```python
from build123d import *

# Parameters (mm, degrees)
SKETCH2_R           = 36.6
SKETCH2_R_2         = 29.45
BOSS_EXTRUDE1_DEPTH = 140
SKETCH3_R           = 36.6
BOSS_EXTRUDE2_DEPTH = 15
SKETCH5_R           = 3.175
CUT_EXTRUDE1_DEPTH  = 52
SKETCH6_R           = 4
SKETCH6_R_2         = 3.175
BOSS_EXTRUDE4_DEPTH = 52
SKETCH7_R           = 3.175
CUT_EXTRUDE2_DEPTH  = 52
SKETCH8_R           = 4
SKETCH8_R_2         = 3.175
BOSS_EXTRUDE5_DEPTH = 10
SKETCH4_R           = 36.6
BOSS_EXTRUDE3_DEPTH = 15


with BuildPart() as part:
    # Sketch2 → Boss-Extrude1 (new body, symmetric)
    with BuildSketch(Plane(origin=(0, 0, 0), x_dir=(1, 0, 0), z_dir=(0, 1, 0))):
        Circle(SKETCH2_R)
        Circle(SKETCH2_R_2, mode=Mode.SUBTRACT)
    extrude(amount=BOSS_EXTRUDE1_DEPTH, both=True)

    # Sketch3 → Boss-Extrude2 (add)
    with BuildSketch(Plane(origin=(0, 140, 0), x_dir=(1, 0, 0), z_dir=(0, 1, 0))):
        Circle(SKETCH3_R)
    extrude(amount=BOSS_EXTRUDE2_DEPTH)

    # Sketch5 → Cut-Extrude1 (cut)
    with BuildSketch(Plane.XY):
        with Locations((0, -117.704465643)):
            Circle(SKETCH5_R)
    extrude(amount=CUT_EXTRUDE1_DEPTH, mode=Mode.SUBTRACT)

    # Sketch6 → Boss-Extrude4 (add)
    with BuildSketch(Plane.XY):
        with Locations((0, -117.704465643)):
            Circle(SKETCH6_R)
        with Locations((0, -117.704465643)):
            Circle(SKETCH6_R_2, mode=Mode.SUBTRACT)
    extrude(amount=BOSS_EXTRUDE4_DEPTH)

    # Sketch7 → Cut-Extrude2 (cut)
    with BuildSketch(Plane(origin=(0, 155, 0), x_dir=(1, 0, 0), z_dir=(0, 1, 0))):
        with Locations((0, 20)):
            Circle(SKETCH7_R)
        Circle(SKETCH7_R)
        with Locations((-20, 0)):
            Circle(SKETCH7_R)
        with Locations((20, 0)):
            Circle(SKETCH7_R)
        with Locations((0, -20)):
            Circle(SKETCH7_R)
    extrude(amount=-CUT_EXTRUDE2_DEPTH, mode=Mode.SUBTRACT)

    # Sketch8 → Boss-Extrude5 (add)
    with BuildSketch(Plane(origin=(0, 155, 0), x_dir=(1, 0, 0), z_dir=(0, 1, 0))):
        Circle(SKETCH8_R)
        Circle(SKETCH8_R_2, mode=Mode.SUBTRACT)
        with Locations((0, 20)):
            Circle(SKETCH8_R)
        with Locations((0, 20)):
            Circle(SKETCH8_R_2, mode=Mode.SUBTRACT)
        with Locations((20, 0)):
            Circle(SKETCH8_R)
        with Locations((20, 0)):
            Circle(SKETCH8_R_2, mode=Mode.SUBTRACT)
        with Locations((-20, 0)):
            Circle(SKETCH8_R)
        with Locations((-20, 0)):
            Circle(SKETCH8_R_2, mode=Mode.SUBTRACT)
        with Locations((0, -20)):
            Circle(SKETCH8_R)
        with Locations((0, -20)):
            Circle(SKETCH8_R_2, mode=Mode.SUBTRACT)
    extrude(amount=BOSS_EXTRUDE5_DEPTH)

    # Sketch4 → Boss-Extrude3 (add)
    with BuildSketch(Plane.XZ.offset(140)):
        Circle(SKETCH4_R)
    extrude(amount=BOSS_EXTRUDE3_DEPTH)


solid = part.part
```
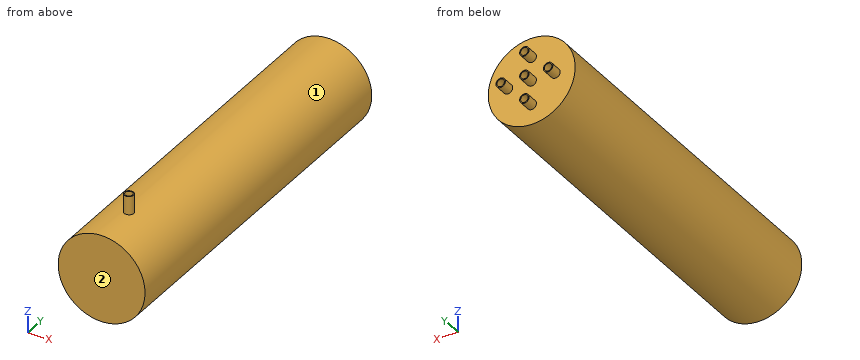
CAD build for the part. Positions are in the model's coordinates, mm. Face numbers are marked on the shaded views. Round coordinates to 2 decimals unless told otherwise and drop trailing zeros. Write each loop counter-clockwise with the first axis right and the second up, starting at its lowest first coordinate (ties: lowest second). Pieces come first, ordered by that corner, then holes. Notation, with made-up numbers: (10.5, -27.5) - (69.5, -27.5) arc R7 ccw to (69.5, -15.5) - close; hole circle Ø10 at (-39, -40). An arc over 180 degrees is marked (long way). Return JSON: item names as keys, results as strings. Group by question number.
Item 1: Probe probe 1 along Z at (x, y) = (0, 151) (3 decimals); probe 2 along Y at (x, z) = (17, 18); probe 3 along Z at (x, y) = (0, 159.5) (3 decimals). List the from-to ranges inside material, lowest first.
Item 2: Mould opens along X. For the marked faces 1 and 2 say: +X half, -X half, draft (parallel to the pull), parting line (faces both ways), or undercut.
Item 3: Band-saw the part on A-A on z = 10. List the corners of the cut face in (x, y) (3 decimals), plus the area to 3 significant figures.
Item 4: Flat gauge pins, fed straight in: pin 1 Ø1 at (x, y) = (17, 41) entering from -Z; pin 2 Ø9 at (x, y) = (-0.5, -118) entering from -Z; pin 3 Ø1 at (x, z) = (16.5, -16.5) entering from +Y. Where does each tip first touch, or does it go through?
Item 5: Band-saw the part on D-D on z = -20. List the corners of the cut face in (x, y) (3 decimals).
Item 6: Band-saw the part on C-C on y = -20.5. List the corners of the cut face in (x, z), plus the area to 3 significant figures.
Item 7: Band-saw the part on B-B on x = -20. List the corners of the cut face in (y, z) (3 decimals), plus the area to 3 significant figures.
Resolved:
{
 "1": {"probe 1": "z = -36.6 to -23.175, -16.825 to -3.175, 3.175 to 16.825, 23.175 to 36.6", "probe 2": "y = -155 to -140, 140 to 155", "probe 3": "z = -24 to -23.175, -16.825 to -16, -4 to -3.175, 3.175 to 4, 16 to 16.825, 23.175 to 24"},
 "2": {"face 1": "parting line", "face 2": "draft"},
 "3": {"outline": "(-35.207, -155) - (35.207, -155) - (35.207, 155) - (-35.207, 155) - close; circle Ø8 at (0, -117.704); hole (-27.7, -140) - (27.7, -140) - (27.7, 140) - (-27.7, 140) - close; hole circle Ø6.35 at (0, -117.704)", "area": "6,340 mm²"},
 "4": {"pin 1": "stops at z = -32.67", "pin 2": "stops at z = -36.6", "pin 3": "stops at y = 155"},
 "5": {"outline": "(-30.652, -155) - (30.652, -155) - (30.652, 155) - (4, 155) - (4, 165) - (3.175, 165) - (3.175, 140) - (21.617, 140) - (21.617, -140) - (-21.617, -140) - (-21.617, 140) - (-3.175, 140) - (-3.175, 165) - (-4, 165) - (-4, 155) - (-30.652, 155) - close"},
 "6": {"outline": "circle Ø73.2 at (0, 0); hole circle Ø58.9 at (0, 0)", "area": "1,480 mm²"},
 "7": {"outline": "(-155, -30.652) - (155, -30.652) - (155, -4) - (165, -4) - (165, -3.175) - (140, -3.175) - (140, -21.617) - (-140, -21.617) - (-140, 21.617) - (140, 21.617) - (140, 3.175) - (165, 3.175) - (165, 4) - (155, 4) - (155, 30.652) - (-155, 30.652) - close", "area": "6,820 mm²"}
}
